Part model, mm, in its own coordinate system. A direction names the side the tool comes from. Give positions to 0.01 mm unless a question says otherwise; leave off trailing zeros. Order: outer loops, then holes, each group sorted by start corner. A loop starts at its lowest first (then second) coordinate and runs counter-clockwise, first axis right, second up. Notation, with made-up numbers: (49, 71.5) - (54, 71.5) arc R33 cw to (54, 106.5) - close; hole circle Ø3 at (39.25, 27.25). An arc over 180 degrees is marked (long way). Use one line per item in the form item = value. Start each with the question number.
1. Pin check, flat tips, straight feed: P1, Ø12, axis at x = 9.5, y = 2.5, coming from the -Z side; P2, Ø8.5, axis at x = -17, y = -12.5, coming from the +Z side; P3, Ø6, axis at y = -1.5, z = 9, coming from the -X side. Stop position of each tip, or through.
2. Band-saw the part on A-A, the plane x = 0. List the corners of the cut face in (y, z).
3. Drill centre lines: line 1 (Y direction, x = 0, z = 16.5); line 2 (Z direction, x = 42, y = -17.25); line 3 (Y direction, x = 0, z = 8). Where is each one in solid material? Low to high.
4. Band-saw the part on B-B, the plane z = 6.5. State how many separate pieces and enclosed holes the cut face has, plus the area to 3 significant figures.
5. Tool access for faces 4 (the face through (27.92, -5.68, 20.52)), 5 (the face through (22, -19, 13.379)), 6 (the face through (0.1, 30.5, -3.621)), 7 (the face through (-2, 12, -3.621)), 8 (the face through (-31.39, -24.1, -4.02)): list every direction of +Z, -Z, +X, -X, +Y, -Y with a clear straight run to the whole face (end or side of a thin tool).
6. Band-saw the part on D-D, the plane x = -42. List the corners of the cut face in (y, z), plus the area to 3 significant figures.
7. Pull direction Z, two halves, no side cores. Call faces 1 (the face through (-8.73, 10.71, -2.63)), 2 (the face through (-36.6, -22.576, 7.5)), 3 (the face through (-27.36, -5.78, -5.78)): +Z half, -Z half, draft (parallel to the pull), parting line (faces both ways), or undercut.
from build123d import *

# Parameters (mm, degrees)
CROQUIS1_R                 = 4
SALIENTE_EXTRUIR1_DEPTH    = 15
CROQUIS2_R                 = 11
CORTAR_EXTRUIR1_DEPTH      = 3
CROQUIS3_R                 = 5.5
CROQUIS3_R_2               = 4
SALIENTE_EXTRUIR2_DEPTH    = 4
CORTAR_EXTRUIR2_DEPTH      = 36.134373023
CORTAR_EXTRUIR2_DEPTH_BACK = 36.134373023
CROQUIS4_R                 = 2.5
CORTAR_EXTRUIR3_START      = -4.5
CORTAR_EXTRUIR3_DEPTH      = 4.5
CORTAR_EXTRUIR4_START      = -2.5
CROQUIS8_R                 = 5.5
CORTAR_EXTRUIR4_DEPTH      = 2.5
CORTAR_EXTRUIR5_DEPTH      = 34.684924933
CORTAR_EXTRUIR5_DEPTH_BACK = 34.684924933
CORTAR_EXTRUIR6_REACH      = 61.188
CORTAR_EXTRUIR7_DEPTH      = 5
CORTAR_EXTRUIR8_DEPTH      = 1.5
SALIENTE_EXTRUIR3_START    = 1
CROQUIS13_R                = 5.5
CROQUIS13_R_2              = 4
SALIENTE_EXTRUIR3_DEPTH    = 1
SCALE1_SCALE               = 2


with BuildPart() as part:
    # Croquis1 → Saliente-Extruir1 (new body)
    with BuildSketch(Plane.XY):
        with BuildLine():
            Line((27.5, -13.890204062), (-27.5, -13.890204062))
            Line((-27.5, -13.890204062), (-27.5, -8.890204062))
            Line((-27.5, -8.890204062), (-16.496411132, -8.890204062))
            ThreePointArc((-16.496411132, -8.890204062), (-15.125192899, -8.346143813), (-14.5, -7.009964621))
            Line((-14.5, -7.009964621), (-13.974877925, 1.743831875))
            ThreePointArc((-13.974877925, 1.743831875), (0, 14.905507967), (13.974877925, 1.743831875))
            Line((13.974877925, 1.743831875), (14.5, -7.009964621))
            ThreePointArc((14.5, -7.009964621), (15.125192899, -8.346143813), (16.496411132, -8.890204062))
            Line((16.496411132, -8.890204062), (27.5, -8.890204062))
            Line((27.5, -8.890204062), (27.5, -13.890204062))
        make_face()
        with Locations((0, 0.905507967)):
            Circle(CROQUIS1_R, mode=Mode.SUBTRACT)
    extrude(amount=SALIENTE_EXTRUIR1_DEPTH)

    # Croquis2 → Cortar-Extruir1 (cut)
    with BuildSketch(Plane.XY.offset(15)):
        with Locations((0, 0.905507967)):
            Circle(CROQUIS2_R)
    cortar_extruir1 = extrude(amount=-CORTAR_EXTRUIR1_DEPTH, mode=Mode.SUBTRACT)

    # Croquis3 → Saliente-Extruir2 (add)
    with BuildSketch(Plane.XY.offset(12)):
        with Locations((0, 0.905507967)):
            Circle(CROQUIS3_R)
        with Locations((0, 0.905507967)):
            Circle(CROQUIS3_R_2, mode=Mode.SUBTRACT)
    extrude(amount=SALIENTE_EXTRUIR2_DEPTH)

    # Croquis4 → Cortar-Extruir2 (cut, two sides: drawn at the far end of the back side and taken through both)
    with BuildSketch(Plane(origin=(0, 0, 0), x_dir=(1, 0, 0), z_dir=(0, 1, 0)).offset(-CORTAR_EXTRUIR2_DEPTH_BACK)):
        with Locations(Location((-21, -7.5, 0), (0, 0, 270))):
            Circle(CROQUIS4_R)
        with Locations(Location((21, -7.5, 0), (0, 0, 270))):
            Circle(CROQUIS4_R)
    extrude(amount=CORTAR_EXTRUIR2_DEPTH + CORTAR_EXTRUIR2_DEPTH_BACK, mode=Mode.SUBTRACT)

    # Simetría1: Cortar-Extruir1 across plane
    add(cortar_extruir1.mirror(Plane.XY.offset(7.5)), mode=Mode.SUBTRACT)

    # Croquis7 → Cortar-Extruir3 (cut)
    with BuildSketch(Plane.XY.offset(15).offset(CORTAR_EXTRUIR3_START)):
        with BuildLine():
            Line((-13.910933618, -13.890204062), (-13.370245715, -4.876924871))
            ThreePointArc((-13.370245715, -4.876924871), (-13.124159844, -4.599675432), (-12.796571792, -4.773202306))
            ThreePointArc((-12.796571792, -4.773202306), (0, -13.094492033), (12.796571792, -4.773202306))
            ThreePointArc((12.796571792, -4.773202306), (13.124159844, -4.599675432), (13.370245715, -4.876924871))
            Line((13.370245715, -4.876924871), (13.910933618, -13.890204062))
            Line((13.910933618, -13.890204062), (-13.910933618, -13.890204062))
        make_face()
    cortar_extruir3 = extrude(amount=CORTAR_EXTRUIR3_DEPTH, mode=Mode.SUBTRACT)

    # Croquis8 → Cortar-Extruir4 (cut)
    with BuildSketch(Plane.XY.offset(15).offset(CORTAR_EXTRUIR4_START)):
        with BuildLine():
            Line((-13.910933618, -13.890204062), (-12.976672359, 1.683951596))
            ThreePointArc((-12.976672359, 1.683951596), (0, 13.905507967), (12.976672359, 1.683951596))
            Line((12.976672359, 1.683951596), (13.910933618, -13.890204062))
            Line((13.910933618, -13.890204062), (-13.910933618, -13.890204062))
        make_face()
        with Locations((0, 0.905507967)):
            Circle(CROQUIS8_R, mode=Mode.SUBTRACT)
    cortar_extruir4 = extrude(amount=CORTAR_EXTRUIR4_DEPTH, mode=Mode.SUBTRACT)

    # Croquis9 → Cortar-Extruir5 (cut, two sides: drawn at the far end of the back side and taken through both)
    with BuildSketch(Plane.XY.offset(12.5).offset(-CORTAR_EXTRUIR5_DEPTH_BACK)):
        Polygon((13.910933618, -13.890204062), (13.861404459, -13.064551894), (-13.861404459, -13.064551894), (-13.910933618, -13.890204062), align=None)
    extrude(amount=CORTAR_EXTRUIR5_DEPTH + CORTAR_EXTRUIR5_DEPTH_BACK, mode=Mode.SUBTRACT)

    # Croquis10 → Cortar-Extruir6 (cut, up to next)
    with BuildSketch(Plane(origin=(27.5, 0, 0), x_dir=(0, 0, -1), z_dir=(1, 0, 0)), mode=Mode.PRIVATE) as cortar_extruir6_sk1:
        Polygon((-15, 15.98971015), (-13, 14.905507967), (-13, 1.743831875), (-15, -8.890204062), align=None)
    cortar_extruir6_tool1 = extrude(cortar_extruir6_sk1.sketch, amount=-CORTAR_EXTRUIR6_REACH, mode=Mode.PRIVATE) & part.part
    # Croquis10 → Cortar-Extruir6 (cut, up to next)
    with BuildSketch(Plane(origin=(27.5, 0, 0), x_dir=(0, 0, -1), z_dir=(1, 0, 0)), mode=Mode.PRIVATE) as cortar_extruir6_sk2:
        Polygon((-2, 14.905507967), (0, 15.98971015), (0, -8.890204062), (-2, 1.743831875), align=None)
    cortar_extruir6_tool2 = extrude(cortar_extruir6_sk2.sketch, amount=-CORTAR_EXTRUIR6_REACH, mode=Mode.PRIVATE) & part.part
    add(cortar_extruir6_tool1.solids().sort_by_distance((27.5, 5.692069, 14.102679))[0], mode=Mode.SUBTRACT)
    add(cortar_extruir6_tool2.solids().sort_by_distance((27.5, 5.692069, 0.897321))[0], mode=Mode.SUBTRACT)

    # Croquis11 → Cortar-Extruir7 (cut)
    with BuildSketch(Plane.XZ.offset(13.890204062)):
        with BuildLine():
            Line((-26.292893219, 14.707106781), (-27.207106781, 13.792893219))
            ThreePointArc((-27.207106781, 13.792893219), (-27.423879533, 13.46846987), (-27.5, 13.085786438))
            Line((-27.5, 13.085786438), (-27.5, 1.914213562))
            ThreePointArc((-27.5, 1.914213562), (-27.423879533, 1.53153013), (-27.207106781, 1.207106781))
            Line((-27.207106781, 1.207106781), (-26.292893219, 0.292893219))
            ThreePointArc((-26.292893219, 0.292893219), (-25.96846987, 0.076120467), (-25.585786438, 0))
            Line((-25.585786438, 0), (-15.540514777, 0))
            Line((-15.540514777, 0), (-15.540514777, -5.530731653))
            Line((-15.540514777, -5.530731653), (-33.970258, -5.530731653))
            Line((-33.970258, -5.530731653), (-33.970258, 16.269467594))
            Line((-33.970258, 16.269467594), (-15.540514777, 16.269467594))
            Line((-15.540514777, 16.269467594), (-15.540514777, 15))
            Line((-15.540514777, 15), (-25.585786438, 15))
            ThreePointArc((-25.585786438, 15), (-25.96846987, 14.923879533), (-26.292893219, 14.707106781))
        make_face()
    cortar_extruir7 = extrude(amount=-CORTAR_EXTRUIR7_DEPTH, mode=Mode.SUBTRACT)

    # Croquis12 → Cortar-Extruir8 (cut)
    with BuildSketch(Plane.XZ.offset(13.890204062)):
        with BuildLine():
            Line((-25, 13.5), (-16.410933618, 13.5))
            ThreePointArc((-16.410933618, 13.5), (-15.703826837, 13.207106781), (-15.410933618, 12.5))
            Line((-15.410933618, 12.5), (-15.410933618, 2.5))
            ThreePointArc((-15.410933618, 2.5), (-15.703826837, 1.792893219), (-16.410933618, 1.5))
            Line((-16.410933618, 1.5), (-25, 1.5))
            ThreePointArc((-25, 1.5), (-25.707106781, 1.792893219), (-26, 2.5))
            Line((-26, 2.5), (-26, 12.5))
            ThreePointArc((-26, 12.5), (-25.707106781, 13.207106781), (-25, 13.5))
        make_face()
    cortar_extruir8 = extrude(amount=-CORTAR_EXTRUIR8_DEPTH, mode=Mode.SUBTRACT)

    # Simetría2: Cortar-Extruir7, Cortar-Extruir8 across plane
    add(cortar_extruir7.mirror(Plane(origin=(0, 0, 0), x_dir=(0, 0, 1), z_dir=(1, 0, 0))), mode=Mode.SUBTRACT)
    add(cortar_extruir8.mirror(Plane(origin=(0, 0, 0), x_dir=(0, 0, 1), z_dir=(1, 0, 0))), mode=Mode.SUBTRACT)

    # Simetría4: Cortar-Extruir3, Cortar-Extruir4 across plane
    add(cortar_extruir3.mirror(Plane.XY.offset(7.5)), mode=Mode.SUBTRACT)
    add(cortar_extruir4.mirror(Plane.XY.offset(7.5)), mode=Mode.SUBTRACT)

    # Croquis13 → Saliente-Extruir3 (add)
    with BuildSketch(Plane(origin=(0, 0, 3), x_dir=(-1, 0, 0), z_dir=(0, 0, -1)).offset(SALIENTE_EXTRUIR3_START)):
        with Locations(Location((0, 0.905507967, 0), (0, 0, 180))):
            Circle(CROQUIS13_R)
        with Locations(Location((0, 0.905507967, 0), (0, 0, 270))):
            Circle(CROQUIS13_R_2, mode=Mode.SUBTRACT)
    extrude(amount=-SALIENTE_EXTRUIR3_DEPTH)


with BuildPart() as part_1:
    # Scale1: scaled about (0, -2.204708481, 7.62083442)
    add(part.part.scale(SCALE1_SCALE).moved(Location((0, 2.204708481, -7.62083442))))


solid = part_1.part
From the geometry:
q1.P1 = -3.62
q1.P2 = 17.38
q1.P3 = -28.56
q2.outline = (-23.92, -2.62) - (-17.98, -2.62) - (-17.98, -1.62) - (-6.98, -1.62) - (-6.98, -3.62) - (-3.98, -3.62) - (-3.98, 24.38) - (-6.98, 24.38) - (-6.98, 16.38) - (-17.98, 16.38) - (-17.98, 17.38) - (-23.92, 17.38) - close; (12.02, -3.62) - (15.02, -3.62) - (15.02, -1.62) - (26.02, -1.62) - (26.02, -2.62) - (30.02, -2.62) - (30.02, -3.62) - (32.02, -3.62) - (32.02, 18.38) - (30.02, 18.38) - (30.02, 17.38) - (26.02, 17.38) - (26.02, 16.38) - (15.02, 16.38) - (15.02, 24.38) - (12.02, 24.38) - close
q3.line_1 = -23.92 to -17.98, -6.98 to -3.98, 12.02 to 15.02, 26.02 to 32.02
q3.line_2 = -7.62 to 2.38, 12.38 to 22.38
q3.line_3 = -23.92 to -3.98, 12.02 to 32.02
q4.separate_pieces = 3
q4.enclosed_holes = 1
q4.area = 2,900 mm²
q5.face_4 = +Z, +X, +Y
q5.face_5 = +Z, -Y
q5.face_6 = -Z, +X, -X, +Y
q5.face_7 = -Z, +Y, -Y
q5.face_8 = -Y
q6.outline = (-25.58, -7.62) - (-15.58, -7.62) - (-15.58, 2.38) - (-22.58, 2.38) - (-22.58, -4.62) - (-25.58, -4.62) - close; (-25.58, 19.38) - (-22.58, 19.38) - (-22.58, 12.38) - (-15.58, 12.38) - (-15.58, 22.38) - (-25.58, 22.38) - close
q6.area = 158 mm²
q7.face_1 = draft
q7.face_2 = undercut
q7.face_3 = -Z half
